Model file for the job. Use its own axes, mm. Coordinates: 2 decimals unless noted, no trailing zeros. Write item = value, one per line. Start each with the question number.
Q1. Flat gauge pins, fed straight in: pin 1 (4 mm diameter, centred on x = 359, y = 533.5, fed in from -Z); pin 2 (5 mm diameter, centred on x = 378, y = 536, fed in from -Z). Where does each tip first touch, or does it go through?
Q2. Mould opens along Y. For faces 1 (the face through (381.308, 534.965, -0.695)), 2 (the face through (349.34, 524.87, 7.35)), 3 (the face through (350.189, 528.845, 2.755)) say: +Y half, -Y half, draft (parallel to the pull), parting line (faces both ways), or undercut.
Q3. Wall check: line 1 (Z direction, x = 372, y = 533.5); line 2 (Z direction, x = 369, y = 532.25); line 3 (X direction, y = 527, z = -9). Give the ranges that are in metal, low to high. Write a range as from..to.
from build123d import *

# Parameters (mm, degrees)
SK_BOLAS_R = 2.0000000000000018


with BuildPart() as part:
    # Sk_Jaula → Jaula (revolve)
    with BuildSketch(Plane.XY, mode=Mode.PRIVATE) as jaula_sk:
        Polygon((380.26368558200323, 538.3272855976807), (383.50631412034375, 539.3497141586763), (384.70917125092683, 535.5348570547463), (381.4665427125863, 534.5124284937507), align=None)
    revolve(jaula_sk.sketch.rotate(Axis((363.69142860825076, 538.3445713117901, 0), (0.3007142826457713, -0.9537142759825079, 0)), 180), axis=Axis((363.69142860825076, 538.3445713117901, 0), (0.3007142826457713, -0.9537142759825079, 0)))

    # Sk_Bolas → Bolas (revolve)
    with BuildSketch(Plane.XY, mode=Mode.PRIVATE) as bolas_sk:
        with Locations((382.486428416465, 536.9310713262134)):
            Circle(SK_BOLAS_R)
    revolve(bolas_sk.sketch.rotate(Axis((362.7892857603134, 541.2057141397376, 0), (0.3007142826457754, -0.9537142759825067, 0)), 180), axis=Axis((362.7892857603134, 541.2057141397376, 0), (0.3007142826457754, -0.9537142759825067, 0)))


solid = part.part
Here are the results:
q1.pin_1 = -18.53
q1.pin_2 = -16.45
q2.face_1 = undercut
q2.face_2 = undercut
q2.face_3 = +Y half
q3.line_1 = -18.39..-14.09, 14.09..18.39
q3.line_2 = -19.19..-15.2, 15.2..19.19
q3.line_3 = 349.22..353.8
